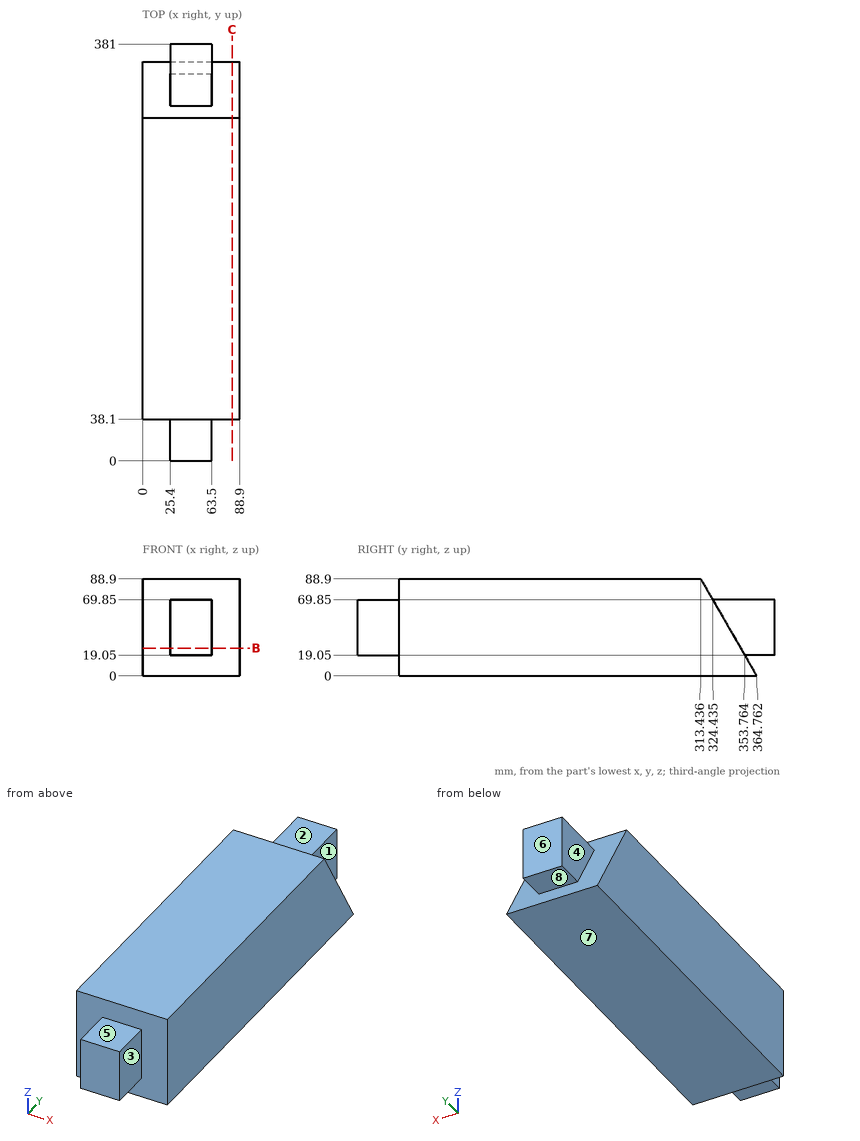
For this review, use the dimensioned drawing (mm, ordinates from the lowest corner) and the shaded views. A direction names the side the tool comes from. Round coordinates to 2 decimals unless told otherwise and drop trailing zeros. Write each loop counter-clockwise with the first axis right and the second up, starting at its lowest first coordinate (ties: lowest second). Pieces come first, ordered by that corner, then holes. Notation, with made-up numbers: (15, 23) -> (68, 23) arc R21 cw to (68, 35) -> close; hole circle Ø5 at (26.25, 53.25). An arc over 180 degrees is marked (long way). Use one line per item in the form item = value.
Q1. Clearance check with flat-ended pins moving along their axes: pin 1 Ø13.5 at (x, y) = (40.5, 372.5) entering from -Z; pin 2 Ø19 at (x, y) = (50.5, 12.5) entering from +Z; pin 3 Ø2 at (x, z) = (42.5, 36.5) entering from -Y; pin 4 Ø4 at (x, z) = (72.5, 17) entering from -Y. State where each tip first meets the part, or that it passes through.
Resolved:
pin_1 = 19.05
pin_2 = 69.85
pin_3 = 0
pin_4 = 38.1
Q2. Consider section C-C (x = 82). State the section outline as (y, z) points.
Resolved:
outline = (38.1, 0) -> (364.76, 0) -> (313.44, 88.9) -> (38.1, 88.9) -> close
Q3. Machinability: for the marked faces 1, 2, 3 and 4, which of the approach directions +Z, -Z, +X, -X, +Y, -Y give a long, thin tool a straight path to every point of the face, cutting with its end or side? Answer none if there is none.
Resolved:
face_1 = +Z, +X, +Y
face_2 = +Z, +X, -X, +Y
face_3 = +Z, -Z, +X, -Y
face_4 = +Z, -X, +Y
Q4. The part is to be moulded in two halves that separate along Z. For the marked faces 5, 6, 7 and 8, say which applies: released by +Z, released by -Z, zero draft, split by the parting line, or undercut.
Resolved:
face_5 = released by +Z
face_6 = zero draft
face_7 = released by -Z
face_8 = undercut
Q5. To check wall thickness, follow probe 1 along X at (y, z) = (359.5, 39); probe 2 along Z at (x, y) = (59.5, 328); probe 3 along Y at (x, z) = (66.5, 60). State the ranges of each line that lie inside material, in increasing order. Write a range as from..to.
Resolved:
probe_1 = 25.4..63.5
probe_2 = 0..69.85
probe_3 = 38.1..330.12
Q6. Consider section B-B (z = 25.5). State the section outline as (x, y) points.
Resolved:
outline = (0, 38.1) -> (25.4, 38.1) -> (25.4, 0) -> (63.5, 0) -> (63.5, 38.1) -> (88.9, 38.1) -> (88.9, 350.04) -> (63.5, 350.04) -> (63.5, 381) -> (25.4, 381) -> (25.4, 350.04) -> (0, 350.04) -> close
